```python
from build123d import *

# Parameters (mm, degrees)
F0_W     = 10
F0_H     = 18.0418604054
F0_H_2   = 25
F0_H_3   = 6.9581395946
F3_R     = 10
F4_DEPTH = 141.6
F5_R     = 1
F6_SIZE2 = 0.99999
F6_SIZE  = 9.99999
F8_D     = 3
F9_D     = 3


# Not quite as in the source:
# - a fillet or chamfer is up to 0.001 mm smaller than in the source, because OpenCascade refuses the exact size


with BuildPart() as f1:
    # F0 (on Front) → F1 (revolve)
    with BuildSketch(Plane.XZ):
        Polygon((-72.5, 15), (-72.5, 0), (0, 0), (0, 25), (-64.5, 25), (-64.5, 15), align=None)
    revolve(axis=Axis((0, 0, 12.5), (0, 0, 1)))

    # F0 (on Front) → F2 (revolve, cut)
    with BuildSketch(Plane.XZ):
        with Locations((5, 34.0209302027)):
            Rectangle(F0_W, F0_H)
        with Locations((5, 12.5)):
            Rectangle(F0_W, F0_H_2)
        with Locations((5, -3.4790697973)):
            Rectangle(F0_W, F0_H_3)
    revolve(axis=Axis((0, 0, 18.0418604054), (0, 0, 1)), mode=Mode.SUBTRACT)

    # F3 (on Front) → F4 (cut)
    with BuildSketch(Plane.XZ):
        Circle(F3_R)
    extrude(amount=-F4_DEPTH, mode=Mode.SUBTRACT)

    # F5
    f5_edges = [f1.edges().sort_by_distance(p)[0] for p in [
        (72.5, 0, 15),
    ]]
    fillet(f5_edges, radius=F5_R)

    # F6 (size 10 and 1 in the source; OpenCascade refuses exactly that, so slightly less here)
    f6_edges = [f1.edges().sort_by_distance(p)[0] for p in [
        (64.5, 0, 25),
    ]]
    chamfer(f6_edges, length=F6_SIZE, length2=F6_SIZE2)

    # F8 (through all)
    with Locations(Plane(origin=(0, 0, 0), x_dir=(1, 0, 0), z_dir=(0, 0, -1))):
        with Locations((24, 0)):
            Hole(F8_D / 2)

    # F9 (through all)
    with Locations(Plane(origin=(0, 0, 0), x_dir=(1, 0, 0), z_dir=(0, 0, -1))):
        with Locations((-24, 0)):
            Hole(F9_D / 2)


solid = f1.part
```
Check sheet for the modelled part. Datum: model origin and axes. Units: mm. A direction names the side the tool comes from. Round coordinates to 2 decimals unless told otherwise and drop trailing zeros. Write each loop counter-clockwise with the first axis right and the second up, starting at its lowest first coordinate (ties: lowest second). Pieces come first, ordered by that corner, then holes. Notation, with made-up numbers: (8.25, 79.5) -> (54.25, 79.5) arc R29 ccw to (54.25, 110.5) -> close; hole circle Ø8 at (-29, -15.5). An arc over 180 degrees is marked (long way). Put each result on its own line as item: value.
(1) Tool access check on faces 1 (the face through (-1, 13, 25)), 2 (the face through (-11, -64, 15)). Record the directions out of +Z, -Z, +X, -X, +Y, -Y that give a thin tool (end or side, any length) a straight path to the whole face; none if there is none.
Values found:
face 1: +Z, +X, -X, +Y, -Y
face 2: +Z
(2) Go/stop test with flat-tipped pins: pin 1 Ø5 at (y, z) = (-25, 8) entering from -X; pin 2 Ø3 at (x, z) = (46.5, 4) entering from +Y; pin 3 Ø3 at (x, z) = (-38.5, 10) entering from +Y; pin 4 Ø2.5 at (x, y) = (24, 0) entering from -Z. Record where each tip stops, or that it passes through.
Values found:
pin 1: stops at x = -68.92
pin 2: stops at y = 56.84
pin 3: stops at y = 62.35
pin 4: passes through
(3) Sectioned sample at B-B (z = 3.5). Enter the section's corners in (x, y), plus the area to 3 significant figures.
Values found:
outline: (-9.37, 3.5) -> (-9.37, 71.89) arc R72.5 ccw (long way) to (9.37, 71.89) -> (9.37, 3.5) arc R10 cw (long way) to start; hole circle Ø3 at (-24, 0); hole circle Ø3 at (24, 0)
area: 15,000 mm^2
(4) Material ranges on line 1 (Z direction, x = 54.5, y = 35); line 2 (X direction, y = 33, z = 1.25); line 3 (Y direction, x = -11, z = 14.5), recorded low to high.
Values found:
line 1: z = 0 to 15
line 2: x = -64.55 to -9.92, 9.92 to 64.55
line 3: y = -71.53 to 71.53
(5) Mould release check, pull along X, two halves, no side actions. Record for faces 3 (the face through (-15, -1, 0)), 4 (the face through (0, 36, 10)), 5 (the face through (-2.17, -9.76, 12.67)), 6 (the face through (-29.32, 56.38, 24.51)): released by +X, released by -X, zero draft, split by the parting line, or undercut.
Values found:
face 3: zero draft
face 4: undercut
face 5: undercut
face 6: split by the parting line
